Read the model definition and answer for the solid it produces. Units are mm, in the model's axes. A direction names the side the tool comes from. Coordinates: 2 decimals unless noted, no trailing zeros. Order: outer loops, then holes, each group sorted by start corner. A loop starts at its lowest first (then second) coordinate and runs counter-clockwise, first axis right, second up. Notation, with made-up numbers: (-31.5, -24.5) -> (10.5, -24.5) arc R29 cw to (10.5, 8.5) -> close; hole circle Ø11 at (-21.5, 35). An arc over 180 degrees is marked (long way). Answer as a JSON object with one key per item and string values. Group by question number.
1) Given pin 1 (0.6 mm diameter, centred on x = 30, z = 1.5, fed in from +Y); pin 2 (1 mm diameter, centred on x = 43, y = 8.5, fed in from +Z), each flat-ended and moving along its own axis, determine where each tip first touches the part or whether it passes through.
2) Section A-A on x = 32 is taken. Determine the outline of the cut face in (y, z), and give its area (3 significant figures).
3) Determine the mould class of faces 1 (the flat face through (47, 4, 2)), 2 (the flat face through (16, 11, 1.5)) for opening direction X: released by +X, released by -X, zero draft, split by the parting line, or undercut.
4) Consider L1, parallel to Y at x = 26, z = 1.75; L2, parallel to X at y = 19.5, z = 1.1; L3, parallel to Y at x = 26.5, z = 1.95. Determine where each line is inside the solid, lowest interval first.
5) Section B-B on x = 47.5 is taken. Determine the outline of the cut face in (y, z), and give its area (3 significant figures).
6) A tool of negligible diameter and unlimited length cuts with its end or side. For faces 3 (the flat face through (38, 11, 0)), 4 (the flat face through (56, 11, 1.5)), from which of +Z, -Z, +X, -X, +Y, -Y can it reach the whole face along a straight path? Write none if from no direction.
from build123d import *

# Parameters (mm, degrees)
SKETCH_W            = 78
SKETCH_H            = 21
PAD_DEPTH           = 1
SKETCH001_W         = 77
SKETCH001_H         = 19
PAD001_DEPTH        = 1
SKETCH002_W         = 2
SKETCH002_H         = 12
POCKET_DEPTH        = 0.5
LINEARPATTERN_COUNT = 17
LINEARPATTERN_PITCH = 4.4375


with BuildPart() as part:
    # Sketch → Pad (new body)
    with BuildSketch(Plane.XY):
        with Locations((39, 10.5)):
            Rectangle(SKETCH_W, SKETCH_H)
    extrude(amount=PAD_DEPTH)

    # Sketch001 (on Face6 of Pad) → Pad001 (join)
    with BuildSketch(Plane.XY.offset(1)):
        with Locations((38.5, 10.5)):
            Rectangle(SKETCH001_W, SKETCH001_H)
    extrude(amount=PAD001_DEPTH)

    # Sketch002 (on Face11 of Pad001) → Pocket (cut)
    with BuildSketch(Plane.XY.offset(2)):
        with Locations((3, 10.5)):
            Rectangle(SKETCH002_W, SKETCH002_H)
    pocket = extrude(amount=-POCKET_DEPTH, mode=Mode.SUBTRACT)

    # LinearPattern: Pocket ×17
    with Locations(*[(i * LINEARPATTERN_PITCH, 0, 0) for i in range(1, LINEARPATTERN_COUNT)]):
        add(pocket, mode=Mode.SUBTRACT)


solid = part.part
Worked answers:
{
 "1": {"pin 1": "stops at y = 20", "pin 2": "stops at z = 1.5"},
 "2": {"outline": "(0, 0) -> (21, 0) -> (21, 1) -> (20, 1) -> (20, 2) -> (1, 2) -> (1, 1) -> (0, 1) -> close", "area": "40.0 mm²"},
 "3": {"face 1": "zero draft", "face 2": "undercut"},
 "4": {"L1": "y = 1 to 4.5, 16.5 to 20", "L2": "x = 0 to 77", "L3": "y = 1 to 20"},
 "5": {"outline": "(0, 0) -> (21, 0) -> (21, 1) -> (20, 1) -> (20, 2) -> (16.5, 2) -> (16.5, 1.5) -> (4.5, 1.5) -> (4.5, 2) -> (1, 2) -> (1, 1) -> (0, 1) -> close", "area": "34.0 mm²"},
 "6": {"face 3": "-Z, +X, -X, +Y, -Y", "face 4": "+Z"}
}
